from build123d import *

# Parameters (mm, degrees)
F0_W     = 64.9
F0_H     = 46.6
F0_W_2   = 63.3
F0_H_2   = 45
F1_DEPTH = 0.8
F2_DEPTH = 14.8
F3_W     = 64.9
F3_H     = 46.6
F3_W_2   = 63.3
F3_H_2   = 45
F4_DEPTH = 0.8
F5_DEPTH = 0.8


with BuildPart() as f1:
    # F0 (on Top) → F1 (new body)
    with BuildSketch(Plane.XY):
        with Locations((-30.4580235958, -37.7106211)):
            Rectangle(F0_W, F0_H)
        with Locations((-30.4580235958, -37.7106211)):
            Rectangle(F0_W_2, F0_H_2, mode=Mode.SUBTRACT)
        with Locations((-30.4580235958, -37.7106211)):
            Rectangle(F0_W_2, F0_H_2)
    extrude(amount=-F1_DEPTH)

    # F0 (on Top) → F2 (join)
    with BuildSketch(Plane.XY):
        with Locations((-30.4580235958, -37.7106211)):
            Rectangle(F0_W, F0_H)
        with Locations((-30.4580235958, -37.7106211)):
            Rectangle(F0_W_2, F0_H_2, mode=Mode.SUBTRACT)
    extrude(amount=F2_DEPTH)

    # F3 (on face) → F4 (join)
    with BuildSketch(Plane.XY.offset(14.8)):
        with Locations((-30.4580235958, -37.7106211)):
            Rectangle(F3_W, F3_H)
        with Locations((-30.4580235958, -37.7106211)):
            Rectangle(F3_W_2, F3_H_2, mode=Mode.SUBTRACT)
        with Locations((-30.4580235958, -37.7106211)):
            Rectangle(F3_W_2, F3_H_2)
    extrude(amount=F4_DEPTH)

    # F5 (cut): a face of the model
    f5_faces = [f1.faces().sort_by_distance(p)[0] for p in [
        (1.9919764042, -37.7106211, 7.4),
    ]]
    extrude(f5_faces, amount=-F5_DEPTH, mode=Mode.SUBTRACT)


solid = f1.part
CAD build for the part. Positions are in the model's coordinates, mm. A direction names the side the tool comes from. Round coordinates to 2 decimals unless told otherwise and drop trailing zeros. Write each loop counter-clockwise with the first axis right and the second up, starting at its lowest first coordinate (ties: lowest second). Pieces come first, ordered by that corner, then holes. Notation, with made-up numbers: M -27.5,-15 L -5.5,-15 A12 cw -5.5,-4 Z; hole C 52.5,48 d2. An arc over 180 degrees is marked long. Put each result on its own line as item: value. Start each with the question number.
1) Drill centre lines: probe 1 along Z at (x, y) = (-53, -38); probe 2 along Y at (x, z) = (-40.5, 2.5); probe 3 along X at (y, z) = (-58, 0.5). Where is each one in solid material? Low to high. Write a range as [from, to].
2) Pin check, flat tip, straight feed: pin 1 Ø2 at (y, z) = (-56, 12.5) entering from +X. Stop position of the tip, or through.
3) Saw through at B-B, the plane y = -21.5. Write the cut outline in (x, z).
4) Pull direction Y, two halves, no side cores. Call faces 3 (the flat face through (-31, -14.411, 7)), 4 (the flat face through (-31, -61.011, 7)), 5 (the flat face through (-31, -37, 0)): pulls with the +Y half, pulls with the -Y half, needs draft (parallel to the pull), parting line crosses it, or undercut.
5) Saw through at A-A, the plane x = -30. Write the cut outline in (y, z).
6) 3-axis set-ups, long thin cutter, end or side, ignore diameter. For faces 1 (the flat face through (-62.908, -38, 7)), 2 (the flat face through (-31, -37, 14.8)): which of +Z, -Z, +X, -X, +Y, -Y reach the whole face in a straight line?
7) Saw through at C-C, the plane z = 2. Write the cut outline in (x, y).
Resolved:
1. probe 1: [-0.8, 0], [14.8, 15.6]
1. probe 2: [-61.01, -60.21], [-15.21, -14.41]
1. probe 3: [-62.91, -62.11]
2. pin 1: x = -62.11
3. outline: M -62.91,-0.8 L 1.19,-0.8 L 1.19,0 L -62.11,0 L -62.11,14.8 L 1.19,14.8 L 1.19,15.6 L -62.91,15.6 Z
4. face 3: pulls with the +Y half
4. face 4: pulls with the -Y half
4. face 5: undercut
5. outline: M -61.01,-0.8 L -14.41,-0.8 L -14.41,15.6 L -61.01,15.6 Z; hole M -60.21,0 L -15.21,0 L -15.21,14.8 L -60.21,14.8 Z
6. face 1: +Z, -Z, -X, +Y, -Y
6. face 2: +X
7. outline: M -62.91,-61.01 L 1.19,-61.01 L 1.19,-60.21 L -62.11,-60.21 L -62.11,-15.21 L 1.19,-15.21 L 1.19,-14.41 L -62.91,-14.41 Z
